Design review of the part built by this model. Coordinates are the model's own, in mm. A direction names the side the tool comes from. Round coordinates to 2 decimals unless told otherwise and drop trailing zeros. Use a Markdown table: item, result.
from build123d import *

# Parameters (mm, degrees)
SKETCH_1_W                  = 82
SKETCH_1_H                  = 50
EXTRUDE_1_DEPTH             = 16
CHAMFER_1_SIZE              = 1.5
HOLE_WIZARD_M41_D           = 3.3
HOLE_WIZARD_M41_DEPTH       = 7.008579979
HOLE_WIZARD_M41_CSINK_D     = 4.05
HOLE_WIZARD_M41_CSINK_ANGLE = 90
HOLE_WIZARD_M41_TIP         = 0.991420021


with BuildPart() as part:
    # Эскиз1 → Бобышка-Вытянуть1 (new body)
    with BuildSketch(Plane(origin=(0, 0, 0), x_dir=(1, 0, 0), z_dir=(0, 1, 0))):
        with Locations((41, 25)):
            Rectangle(SKETCH_1_W, SKETCH_1_H)
    extrude(amount=EXTRUDE_1_DEPTH)

    # Фаска1
    chamfer_1_edges = [part.edges().sort_by_distance(p)[0] for p in [
        (82, 16, -25),
        (41, 16, -50),
        (0, 16, -25),
        (41, 16, 0),
    ]]
    chamfer(chamfer_1_edges, length=CHAMFER_1_SIZE)

    # Отверстие обработанное метчиком M41
    with Locations(Plane(origin=(22, 16, -37.5), x_dir=(0, 0, 1), z_dir=(0, 1, 0))):
        with Locations((0, 0), (25, 0), (0, 38), (25, 38)):
            CounterSinkHole(HOLE_WIZARD_M41_D / 2, HOLE_WIZARD_M41_CSINK_D / 2, depth=HOLE_WIZARD_M41_DEPTH, counter_sink_angle=HOLE_WIZARD_M41_CSINK_ANGLE)
            with Locations((0, 0, -(HOLE_WIZARD_M41_DEPTH + HOLE_WIZARD_M41_TIP / 2))):  # 118° drill point
                Cone(0, HOLE_WIZARD_M41_D / 2, HOLE_WIZARD_M41_TIP, mode=Mode.SUBTRACT)


solid = part.part
1. Wall thickness on line 1 along Z through (x, y) = (60, 14); line 2 along X through (y, z) = (11, -37.5); line 3 along Z through (x, y) = (8, 14.75): over which ranges is each line inside the solid? List them lowest first. Write a range as from..to.
Check values:
| item | result |
|---|---|
| line 1 | z = -50..-39.15, -35.85..-14.15, -10.85..0 |
| line 2 | x = 0..20.35, 23.65..58.35, 61.65..82 |
| line 3 | z = -49.75..-0.25 |
2. Machinability: for faces 1 (the face through (40, 0, -25)), 2 (the face through (23.115, 12.262, -36.284)), which of the approach directions +Z, -Z, +X, -X, +Y, -Y give a long, thin tool a straight path to every point of the face, cutting with its end or side? Answer none if there is none.
Check values:
| item | result |
|---|---|
| face 1 | +Z, -Z, +X, -X, -Y |
| face 2 | +Y |
3. The part is to be moulded in two halves that separate along X. For faces 3 (the face through (58.536, 12.262, -13.261)), 4 (the face through (81.2, 15.3, -24.7)), 5 (the face through (40, 16, -25)), say which applies: pulls with the +X half, pulls with the -X half, needs draft (parallel to the pull), parting line crosses it, or undercut.
Check values:
| item | result |
|---|---|
| face 3 | undercut |
| face 4 | pulls with the +X half |
| face 5 | needs draft |
